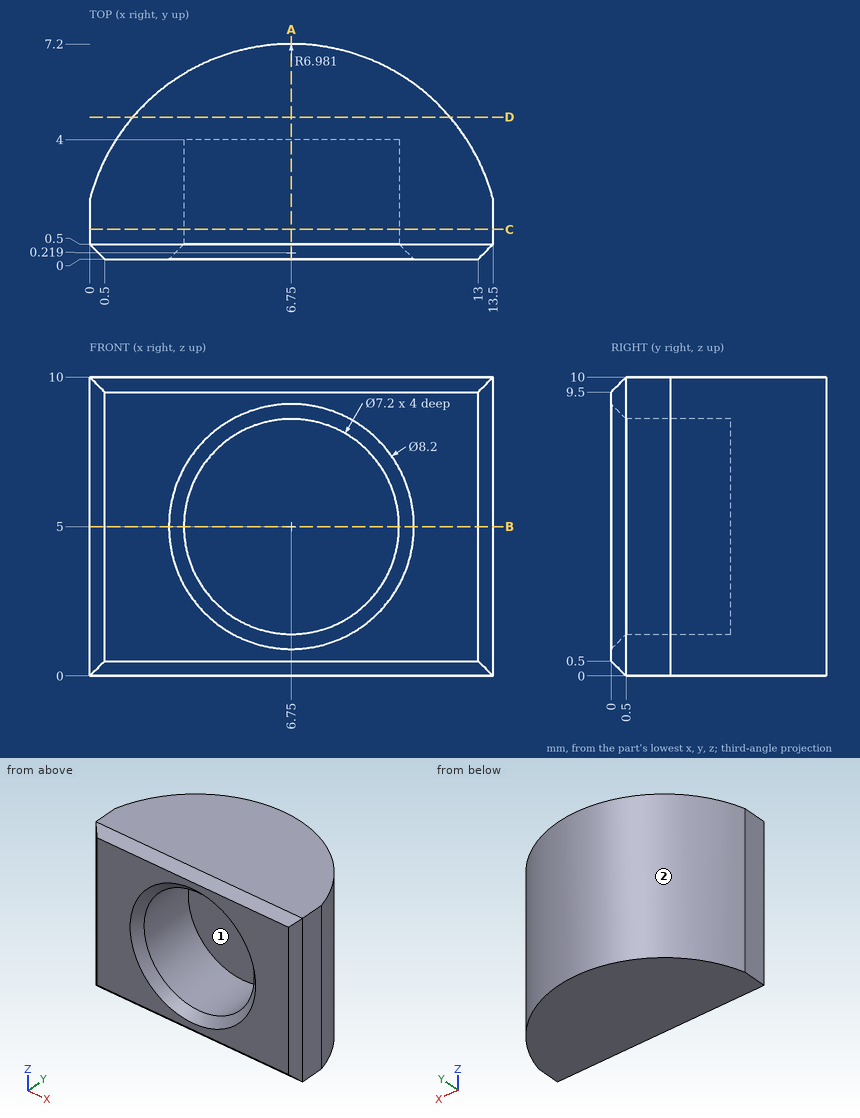
The figure shows three views and two pictorial views of one solid part (mm, origin at its lowest corner). Answer the questions. A direction names the side the tool comes from. Give positions to 0.01 mm unless a question says otherwise; leave off trailing zeros. Order: outer loops, then holes, each group sorted by start corner. A loop starts at its lowest first (then second) coordinate and runs counter-clockwise, first axis right, second up. Notation, with made-up numbers: (0.5, 59) -> (20.5, 59) arc R25 ccw to (20.5, 79) -> close; hole circle Ø11 at (-26, -7). An arc over 180 degrees is marked (long way). One line per item, written item: value.
1) Find section B-B, the plane z = 5. Determine the outline of the cut face in (x, y), plus the area to 3 significant figures.
Reported:
outline: (0, 0.5) -> (0.5, 0) -> (2.65, 0) -> (3.15, 0.5) -> (3.15, 4) -> (10.35, 4) -> (10.35, 0.5) -> (10.85, 0) -> (13, 0) -> (13.5, 0.5) -> (13.5, 2) arc R6.98 ccw to (0, 2) -> close
area: 49.7 mm^2
2) Find the intervals of material crossed by line 1 (X direction, y = 2.45, z = 5); line 2 (Z direction, x = 8.5, y = 2.5); line 3 (Z direction, x = 5.5, y = 1.75), in increasing order.
Reported:
line 1: x = 0.14 to 3.15, 10.35 to 13.36
line 2: z = 0 to 1.85, 8.15 to 10
line 3: z = 0 to 1.62, 8.38 to 10
3) Find section D-D, the plane y = 4.75. Determine the outline of the cut face in (x, z).
Reported:
outline: (1.44, 0) -> (12.06, 0) -> (12.06, 10) -> (1.44, 10) -> close
4) Find section A-A, the plane x = 6.75. Determine the outline of the cut face in (y, z), plus the area to 3 significant figures.
Reported:
outline: (0, 0.5) -> (0.5, 0) -> (7.2, 0) -> (7.2, 10) -> (0.5, 10) -> (0, 9.5) -> (0, 9.1) -> (0.5, 8.6) -> (4, 8.6) -> (4, 1.4) -> (0.5, 1.4) -> (0, 0.9) -> close
area: 42.7 mm^2
5) A tool of negligible diameter and unlimited length cuts with its end or side. For the marked faces 1 and 2, from which of +Z, -Z, +X, -X, +Y, -Y can it reach the whole face along a straight path? Write none if from no direction.
Reported:
face 1: -Y
face 2: +Z, -Z, +Y
6) Find section C-C, the plane y = 1. Determine the outline of the cut face in (x, z), plus the area to 3 significant figures.
Reported:
outline: (0, 0) -> (13.5, 0) -> (13.5, 10) -> (0, 10) -> close; hole circle Ø7.2 at (6.75, 5)
area: 94.3 mm^2
7) A flat-ended cylindrical pin translates along its axis: P1, Ø2, axis at x = 6.5, z = 6.5, coming from the -Y side. Find the tip coordinate at first contact, or state that the pin passes through.
Reported:
P1: stops at y = 4
